Input: part model. Units: mm. Frame: model coordinates. A direction names the side the tool comes from. Round coordinates to 2 decimals unless told otherwise and drop trailing zeros. Order: outer loops, then holes, each group sorted by start corner. A loop starts at its lowest first (then second) coordinate and runs counter-clockwise, first axis right, second up. Notation, with made-up numbers: (21.25, 10.25) -> (28.25, 10.25) arc R27 ccw to (28.25, 26.25) -> close; hole circle Ø10 at (34.25, 19.5). An arc over 180 degrees is marked (long way). Use a Markdown table: item, result.
from build123d import *

# Parameters (mm, degrees)
BOSS_EXTRUDE1_DEPTH = 6.35
FILLET1_R           = 2.54


with BuildPart() as part:
    # Sketch1 → Boss-Extrude1 (new body)
    with BuildSketch(Plane(origin=(0, 0, 0), x_dir=(1, 0, 0), z_dir=(0, 1, 0))):
        with BuildLine():
            Line((0, 50.8), (0, 63.5))
            ThreePointArc((0, 63.5), (31.75, 54.99261314), (54.99261314, 31.75))
            Line((54.99261314, 31.75), (43.994090512, 25.4))
            ThreePointArc((43.994090512, 25.4), (50.8, 0), (43.994090512, -25.4))
            Line((43.994090512, -25.4), (54.99261314, -31.75))
            ThreePointArc((54.99261314, -31.75), (31.75, -54.99261314), (0, -63.5))
            Line((0, -63.5), (0, -50.8))
            ThreePointArc((0, -50.8), (-25.4, -43.994090512), (-43.994090512, -25.4))
            Line((-43.994090512, -25.4), (-54.99261314, -31.75))
            ThreePointArc((-54.99261314, -31.75), (-63.5, 0), (-54.99261314, 31.75))
            Line((-54.99261314, 31.75), (-43.994090512, 25.4))
            ThreePointArc((-43.994090512, 25.4), (-25.4, 43.994090512), (0, 50.8))
        make_face()
        with BuildLine():
            ThreePointArc((-4.50045673, 15.62060899), (-11.494727835, 11.494727835), (-15.62060899, 4.50045673))
            ThreePointArc((-15.62060899, 4.50045673), (-36.8935, 0), (-15.62060899, -4.50045673))
            ThreePointArc((-15.62060899, -4.50045673), (-11.494727835, -11.494727835), (-4.50045673, -15.62060899))
            ThreePointArc((-4.50045673, -15.62060899), (0, -36.8935), (4.50045673, -15.62060899))
            ThreePointArc((4.50045673, -15.62060899), (11.494727835, -11.494727835), (15.62060899, -4.50045673))
            ThreePointArc((15.62060899, -4.50045673), (36.8935, 0), (15.62060899, 4.50045673))
            ThreePointArc((15.62060899, 4.50045673), (11.494727835, 11.494727835), (4.50045673, 15.62060899))
            ThreePointArc((4.50045673, 15.62060899), (0, 36.8935), (-4.50045673, 15.62060899))
        make_face(mode=Mode.SUBTRACT)
    extrude(amount=BOSS_EXTRUDE1_DEPTH)

    # Fillet1
    fillet1_edges = [part.edges().sort_by_distance(p)[0] for p in [
        (4.50045673, 3.175, -15.62060899),
        (-4.50045673, 3.175, -15.62060899),
        (-15.62060899, 3.175, -4.50045673),
        (-15.62060899, 3.175, 4.50045673),
        (-4.50045673, 3.175, 15.62060899),
        (4.50045673, 3.175, 15.62060899),
    ]]
    fillet(fillet1_edges, radius=FILLET1_R)


solid = part.part
1) Cut plane C-C on x = -41. Return loops of the section in (y, z), and give its area (3 significant figures).
Answer key:
| item | result |
|---|---|
| outline | (0, -29.99) -> (6.35, -29.99) -> (6.35, 29.99) -> (0, 29.99) -> close |
| area | 381 mm^2 |
2) Contact query for flat-ended pins moving along their axis: P1, Ø20, axis at x = 25.781, z = 0, coming from the +Y side; P2, Ø3, axis at y = 4, z = -57, coming from the -X side. Output: stop coordinate, or through.
Answer key:
| item | result |
|---|---|
| P1 | passes through |
| P2 | stops at x = 0 |
3) Set-up query: faces 4 (the face through (-11.46, 3.13, -11.53)), 5 (the face through (0, 3, 57)), 6 (the face through (0, 3, -57)), 7 (the face through (49.416, 3.131, 28.531)), 8 (the face through (-63.5, 3.1, 0.5)). Return all of +Z, -Z, +X, -X, +Y, -Y with unobstructed straight access to the full face (end or side cutting, diameter ignored); none if empty.
Answer key:
| item | result |
|---|---|
| face 4 | +Y, -Y |
| face 5 | +Z, -X, +Y, -Y |
| face 6 | -Z, -X, +Y, -Y |
| face 7 | +X, +Y, -Y |
| face 8 | -X, +Y, -Y |
4) Cut plane B-B on x = -5.5. Return loops of the section in (y, z).
Answer key:
| item | result |
|---|---|
| outline | (0, -50.5) -> (6.35, -50.5) -> (6.35, -35.44) -> (0, -35.44) -> close; (0, 35.44) -> (6.35, 35.44) -> (6.35, 50.5) -> (0, 50.5) -> close |
5) Ray query, probe 1 along X at (y, z) = (3, -9); probe 2 along Z at (x, y) = (9.5, 1.5); probe 3 along X at (y, z) = (3, 0). Return the intervals inside material, ascending.
Answer key:
| item | result |
|---|---|
| probe 1 | x = -62.86 to -32.3, -19.26 to -13.54, 13.54 to 19.26, 32.3 to 50 |
| probe 2 | z = -62.79 to -31.55, -20.02 to -13.19, 13.19 to 20.02, 31.55 to 62.79 |
| probe 3 | x = -63.5 to -36.89, 36.89 to 50.8 |
6) Cut plane D-D on z = 39. Return loops of the section in (x, y).
Answer key:
| item | result |
|---|---|
| outline | (-32.55, 0) -> (50.11, 0) -> (50.11, 6.35) -> (-32.55, 6.35) -> close |
7) Cut plane A-A on z = 0. Return loops of the section in (x, y).
Answer key:
| item | result |
|---|---|
| outline | (-63.5, 0) -> (-36.89, 0) -> (-36.89, 6.35) -> (-63.5, 6.35) -> close; (36.89, 0) -> (50.8, 0) -> (50.8, 6.35) -> (36.89, 6.35) -> close |
8) Draft query along Z for faces 1 (the face through (0.366, 3.131, -36.887)), 2 (the face through (-49.57, 3.13, -28.62)), 3 (the face through (-49.416, 3.131, 28.531)). Return one class per face: released by +Z, released by -Z, zero draft, split by the parting line, or undercut.
Answer key:
| item | result |
|---|---|
| face 1 | undercut |
| face 2 | released by -Z |
| face 3 | released by +Z |
